```python
from build123d import *

# Parameters (mm, degrees)
F2_W     = 9.4
F2_H     = 3.02
F3_DEPTH = 20
F4_SIZE  = 0.5


with BuildPart() as f1:
    # F0 (on Front) → F1 (revolve)
    with BuildSketch(Plane.XZ):
        with BuildLine():
            Line((0, 0), (0, 25))
            ThreePointArc((0, 25), (-5.529221, 22.567318), (-7.471553, 16.847389))
            Line((-7.471553, 16.847389), (-6, 0))
            Line((-6, 0), (0, 0))
        make_face()
    revolve(axis=Axis((0, 0, 13.963234), (0, 0, 1)))

    # F2 (on face) → F3 (cut)
    with BuildSketch(Plane(origin=(0, 0, 0), x_dir=(1, 0, 0), z_dir=(0, 0, -1))):
        Rectangle(F2_W, F2_H)
    extrude(amount=-F3_DEPTH, mode=Mode.SUBTRACT)

    # F4
    f4_edges = [f1.edges().sort_by_distance(p)[0] for p in [
        (6, 0, 0),
    ]]
    chamfer(f4_edges, length=F4_SIZE)


solid = f1.part
```
Geometry check sheet. Reference: the model listing, model coordinates, mm. Give positions to 0.01 mm unless a question says otherwise; leave off trailing zeros. Loops run counter-clockwise (first coordinate to the right, second up) from the corner with the lowest first, then second, coordinate; pieces in that order, holes last. Notation, with made-up numbers: M 9.5,-4 L 24.5,-4 A32 cw 24.5,27 Z; hole C 14,55 d3. An arc over 180 degrees is marked long. Write item = value, one per line.
(1) Sectioned sample at A-A, the plane z = 6.25. Record the cut outline in (x, y), plus the area to 3 significant figures.
Answer below:
outline = C 0,0 d13.09; hole M -4.7,-1.51 L 4.7,-1.51 L 4.7,1.51 L -4.7,1.51 Z
area = 106 mm2
(2) Gauge pin test, flat ends, axial feed: pin 1 Ø2.5 at (y, z) = (0, 8) entering from +X; pin 2 Ø7.5 at (x, z) = (-0.5, 10) entering from -Y; pin 3 Ø7.5 at (x, z) = (-0.5, 7.5) entering from +Y. Record the tip position at first contact, or that the pin passes through.
Answer below:
pin_1 = 6.81
pin_2 = -7.2
pin_3 = 6.98
(3) Release check for a two-part mould opening along Y. For faces 1 (the face through (1.463, 6.587, 8.558)), 2 (the face through (4.7, 0, 10)), 3 (the face through (0, 2, 0)) record: released by +Y, released by -Y, zero draft, split by the parting line, or undercut.
Answer below:
face_1 = split by the parting line
face_2 = undercut
face_3 = zero draft
(4) Material ranges on line 1 (Y direction, x = 2, z = 4.75); line 2 (Y direction, x = 0.25, z = 19.75); line 3 (X direction, y = 1.25, z = 19.5), recorded low to high. Write a range as [from, to].
Answer below:
line_1 = [-6.1, -1.51], [1.51, 6.1]
line_2 = [-7.15, -1.51], [1.51, 7.15]
line_3 = [-7.12, -4.7], [4.7, 7.12]
